```python
from build123d import *

# Parameters (mm, degrees)
RESSALTO_EXTRUS_O1_DEPTH                      = 20
ESBO_O2_W                                     = 16
ESBO_O2_H                                     = 16
CORTE_EXTRUS_O1_DEPTH                         = 20
CORTE_EXTRUS_O2_DEPTH                         = 34.120990323
CHANFRO2_SIZE                                 = 1.5
FURO_ROSCADO_DE_M2_51_D                       = 2.05
ESBO_O8_W                                     = 8
ESBO_O8_H                                     = 5
RESSALTO_EXTRUS_O2_DEPTH                      = 12
CHANFRO3_SIZE                                 = 1.5
FURO_ROSCADO_PARA_CONDU_TE_DE_M3X0_51_D       = 3.15
BROCA_DE_ROSQUEAR_PARA_TARRAXA_DE_M2_51_D     = 2.05
BROCA_DE_ROSQUEAR_PARA_TARRAXA_DE_M2_51_DEPTH = 4


with BuildPart() as part:
    # Esboço1 → Ressalto-extrusão1 (new body)
    with BuildSketch(Plane.XY):
        with BuildLine():
            Line((0, 0), (0, 12))
            Line((0, 12), (9.400080843, 20.039805977))
            ThreePointArc((9.400080843, 20.039805977), (13.673368365, 20.633158174), (16, 17))
            Line((16, 17), (16, 4))
            Line((16, 4), (16, 0))
            Line((16, 0), (0, 0))
        make_face()
    extrude(amount=RESSALTO_EXTRUS_O1_DEPTH)

    # Esboço2 → Corte-extrusão1 (cut)
    with BuildSketch(Plane(origin=(16, 0, 0), x_dir=(0, 0, -1), z_dir=(1, 0, 0))):
        with Locations((-8, 13)):
            Rectangle(ESBO_O2_W, ESBO_O2_H)
    extrude(amount=-CORTE_EXTRUS_O1_DEPTH, mode=Mode.SUBTRACT)

    # Esboço3 → Corte-extrusão2 (cut, through all)
    with BuildSketch(Plane.XY.offset(20)):
        Polygon((0, 0), (4, 0), (4, 15.42116461), (0, 12), align=None)
    extrude(amount=-CORTE_EXTRUS_O2_DEPTH, mode=Mode.SUBTRACT)

    # Chanfro2
    chanfro2_edges = [part.edges().sort_by_distance(p)[0] for p in [
        (13.673368365, 20.633158174, 20),
        (6.700040421, 17.730485293, 20),
        (4, 7.710582305, 20),
        (16, 8.5, 20),
    ]]
    chamfer(chanfro2_edges, length=CHANFRO2_SIZE)

    # Furo roscado de M2.51 (through all)
    with Locations(Plane(origin=(12, 17, 20), x_dir=(1, 0, 0), z_dir=(0, 0, 1))):
        with Locations((0, 0)):
            Hole(FURO_ROSCADO_DE_M2_51_D / 2)

    # Esboço8 → Ressalto-extrusão2 (add)
    with BuildSketch(Plane.ZY.offset(-4)):
        with Locations((4, 2.5)):
            Rectangle(ESBO_O8_W, ESBO_O8_H)
    extrude(amount=RESSALTO_EXTRUS_O2_DEPTH)

    # Chanfro3
    chanfro3_edges = [part.edges().sort_by_distance(p)[0] for p in [
        (-2, 5, 8),
        (-8, 2.5, 0),
        (-8, 2.5, 8),
        (-8, 5, 4),
        (4, 5, 0),
        (16, 5, 8),
        (16, 2.5, 0),
        (4, 5, 12),
        (4, 2.5, 8),
    ]]
    chamfer(chanfro3_edges, length=CHANFRO3_SIZE)

    # Furo roscado para conduíte de M3x0.51 (through all)
    with Locations(Plane(origin=(-2, 0, 4), x_dir=(0, 0, -1), z_dir=(0, -1, 0))):
        with Locations((0, 0), (0, 12), (-10, 12)):
            Hole(FURO_ROSCADO_PARA_CONDU_TE_DE_M3X0_51_D / 2)

    # Broca de rosquear para tarraxa de M2.51
    with Locations(Plane(origin=(12, 6, 20), x_dir=(1, 0, 0), z_dir=(0, 0, 1))):
        with Locations((0, 0), (0, 6)):
            Hole(BROCA_DE_ROSQUEAR_PARA_TARRAXA_DE_M2_51_D / 2, depth=BROCA_DE_ROSQUEAR_PARA_TARRAXA_DE_M2_51_DEPTH)


solid = part.part
```
Design review of the part built by this model. Coordinates are the model's own, in mm. A direction names the side the tool comes from. Give positions to 0.01 mm unless a question says otherwise; leave off trailing zeros. Order: outer loops, then holes, each group sorted by start corner. A loop starts at its lowest first (then second) coordinate and runs counter-clockwise, first axis right, second up. Notation, with made-up numbers: (65, -3.5) -> (113, -3.5) arc R19 ccw to (113, 5.5) -> close; hole circle Ø10 at (-7.75, 8.5). An arc over 180 degrees is marked (long way). Write item = value, one per line. Start each with the question number.
(1) For faces 4 (the face through (6, 5, 7)), 5 (the face through (4, 6, 17)), 6 (the face through (15.2, 4.3, 8.9)), list the 3-axis set-ups (+Z, -Z, +X, -X, +Y, -Y) from which the entire face can be reached by the end or side of a thin tool; tool diameter is ignored.
(2) We need section A-A on x = -2. Write out the cut boundary in (y, z) (3 decimals), plus the area to 3 significant figures.
(3) We need section C-C on y = 3. Write out the cut boundary in (x, z) (3 decimals), plus the area to 3 significant figures.
(4) We need section D-D on z = 16.5. Write out the cut boundary in (x, y) (3 decimals), plus the area to 3 significant figures.
(5) To check wall thickness, follow line 1 along Y through (x, z) = (12, 18.5) (3 decimals); line 2 along X through (y, z) = (3.2, 14) (3 decimals); line 3 along Y through (x, z) = (12, 19.15) (3 decimals). State the ranges of each line that lie inside material, in increasing order.
(6) Mouldability with a two-part tool opening along X and no side actions: class faces 1 (the face through (-7, 4, 1)), 2 (the face through (15.3, 8.6, 19.2)), 3 (the face through (-2.96, 2.53, 2.75)) as +X half, -X half, draft (parallel to the pull), parting line (faces both ways), or undercut.
(7) For pin 1 (6 mm diameter, centred on y = 12, z = 13.5, fed in from +X); pin 2 (1.2 mm diameter, centred on x = 12, y = 6, fed in from +Z); pin 3 (8 mm diameter, centred on x = 4, z = 14, fed in from +Y); pin 4 (2.5 mm diameter, centred on y = 4, z = 13, fed in from -X), all flat-tipped, find the tip position at first contact; note any pin that passes through.
(8) We need section B-B on y = 6. Write out the cut boundary in (x, z) (3 decimals).
Numbers:
q1.face_4 = -Z, +X, -X, +Y
q1.face_5 = +Z, -X, +Y, -Y
q1.face_6 = -Z, +X, +Y
q2.outline = (0, 0) -> (3.5, 0) -> (5, 1.5) -> (5, 2.425) -> (0, 2.425) -> close; (0, 5.575) -> (5, 5.575) -> (5, 6.5) -> (3.5, 8) -> (0, 8) -> close
q2.area = 22.0 mm^2
q3.outline = (-8, 1.5) -> (-6.5, 0) -> (14.5, 0) -> (16, 1.5) -> (16, 18.5) -> (14.5, 20) -> (5.5, 20) -> (4, 18.5) -> (4, 9.5) -> (2.5, 8) -> (-6.5, 8) -> (-8, 6.5) -> close; hole circle Ø3.15 at (-2, 4); hole circle Ø3.15 at (10, 4); hole circle Ø3.15 at (10, 14)
q3.area = 308 mm^2
q4.outline = (4, 0) -> (16, 0) -> (16, 17) arc R4 ccw to (9.4, 20.04) -> (4, 15.421) -> close; hole circle Ø2.05 at (12, 6); hole circle Ø2.05 at (12, 12); hole circle Ø2.05 at (12, 17)
q4.area = 220 mm^2
q5.line_1 = 0 to 4.975, 7.025 to 10.975, 13.025 to 15.975, 18.025 to 21
q5.line_2 = 4 to 8.425, 11.575 to 16
q5.line_3 = 0 to 4.975, 7.025 to 10.975, 13.025 to 15.975, 18.025 to 20.35
q6.face_1 = -X half
q6.face_2 = +X half
q6.face_3 = undercut
q7.pin_1 = 16
q7.pin_2 = through
q7.pin_3 = 18.38
q7.pin_4 = 4
q8.outline = (4, 16) -> (10.975, 16) -> (10.975, 20) -> (5.5, 20) -> (4, 18.5) -> close; (13.025, 16) -> (16, 16) -> (16, 18.5) -> (14.5, 20) -> (13.025, 20) -> close
